Design review of the part shown in the three views and the two pictorial views. Dimensions are in mm from the part's minimum x, y and z. A direction names the side the tool comes from. Round coordinates to 2 decimals unless told otherwise and drop trailing zeros. Order: outer loops, then holes, each group sorted by start corner. A loop starts at its lowest first (then second) coordinate and runs counter-clockwise, first axis right, second up.
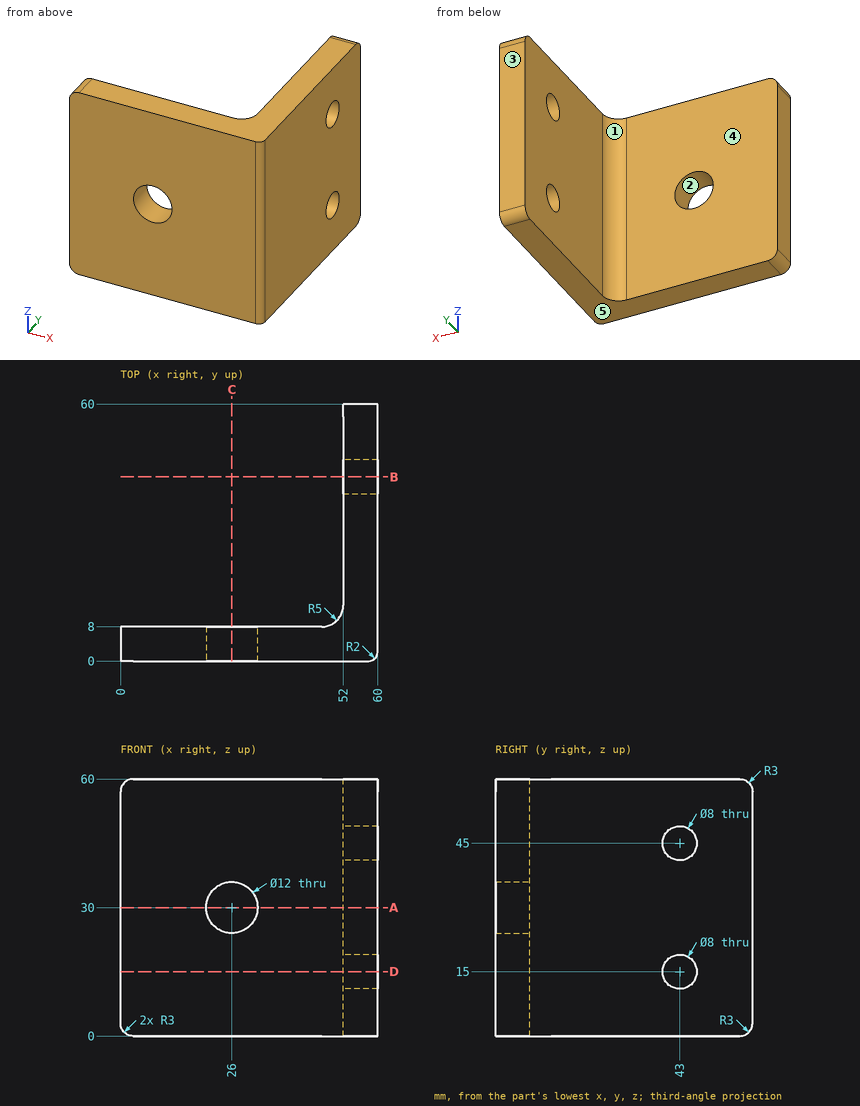
(1) Consider section C-C (x = 26). Write out the cut boundary in (y, z), and give its area (3 significant figures).
Data:
outline: (0, 0) - (8, 0) - (8, 24) - (0, 24) - close; (0, 36) - (8, 36) - (8, 60) - (0, 60) - close
area: 384 mm2
(2) Consider section B-B (y = 43). Write out the cut boundary in (x, z).
Data:
outline: (52, 0) - (60, 0) - (60, 11) - (52, 11) - close; (52, 19) - (60, 19) - (60, 41) - (52, 41) - close; (52, 49) - (60, 49) - (60, 60) - (52, 60) - close
(3) To check wall thickness, follow probe 1 along Z at (x, y) = (55.75, 43); probe 2 along Z at (x, y) = (26, 3.25); probe 3 along X at (y, z) = (36, 30). State the ranges of each line that lie inside material, in increasing order.
Data:
probe 1: z = 0 to 11, 19 to 41, 49 to 60
probe 2: z = 0 to 24, 36 to 60
probe 3: x = 52 to 60
(4) Consider section A-A (z = 30). Write out the cut boundary in (x, y), and give its area (3 significant figures).
Data:
outline: (0, 0) - (20, 0) - (20, 8) - (0, 8) - close; (32, 0) - (58, 0) arc R2 ccw to (60, 2) - (60, 60) - (52, 60) - (52, 13) arc R5 cw to (47, 8) - (32, 8) - close
area: 805 mm2
(5) Consider section D-D (z = 15). Write out the cut boundary in (x, y), and give its area (3 significant figures).
Data:
outline: (0, 0) - (58, 0) arc R2 ccw to (60, 2) - (60, 39) - (52, 39) - (52, 13) arc R5 cw to (47, 8) - (0, 8) - close; (52, 47) - (60, 47) - (60, 60) - (52, 60) - close
area: 837 mm2
(6) Insertion check: pin 1 (6.5 mm diameter, centred on y = 43, z = 45, fed in from +X); pin 2 (10.5 mm diameter, centred on y = 43, z = 15, fed in from -X). Each pin has a flat end and moves straight along its axis. Give the tip position at first contact, or say it passes through.
Data:
pin 1: passes through
pin 2: stops at x = 52
(7) For the marked faces 4 and 5, list the 3-axis set-ups (+Z, -Z, +X, -X, +Y, -Y) from which the entire face can be reached by the end or side of a thin tool; tool diameter is ignored.
Data:
face 4: +Z, -Z, -X, +Y
face 5: -Z, +X, -X, +Y, -Y
(8) Draft analysis for pull direction X (two halves, no side actions). For the marked faces 1, 2 and 3, state which applies: pulls with the +X half, pulls with the -X half, needs draft (parallel to the pull), parting line crosses it, or undercut.
Data:
face 1: pulls with the -X half
face 2: undercut
face 3: needs draft
